Here's how the part is built. I have some questions about the finished solid (model axes, mm). Face numbers are marked on the shaded views. Round coordinates to 2 decimals unless told otherwise and drop trailing zeros. Loops run counter-clockwise (first coordinate to the right, second up) from the corner with the lowest first, then second, coordinate; pieces in that order, holes last. Notation, with made-up numbers: M 67,-23.75 L 100,-23.75 A32 ccw 100,13.25 Z; hole C 30.5,38 d10. An arc over 180 degrees is marked long. Answer as a JSON object with one key per item and string values.
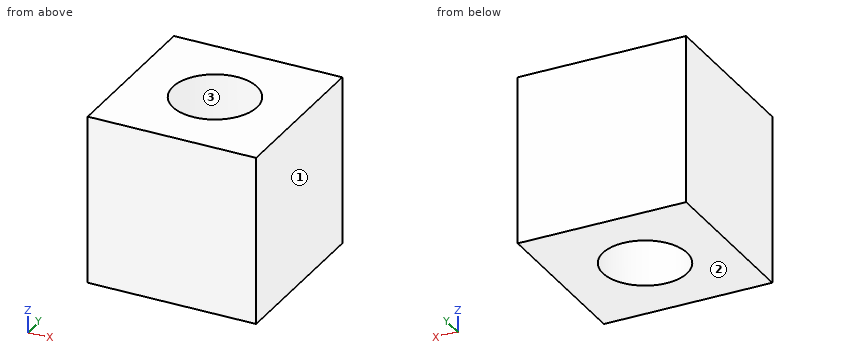
Autodesk Fusion 360 part; units mm, degrees
sketch "WCS Profiles" plane through (0, 0, 0) normal (0, 0, 1) x (1, 0, 0)
  line L0 (20, 20) -> (-20, 20)
  line L1 (-20, 20) -> (-20, -20)
  line L2 (-20, -20) -> (20, -20)
  line L3 (20, -20) -> (20, 20)
  line L4 (20, 20) -> (-20, -20) construction
  line L5 (-20, 20) -> (20, -20) construction
  circle A0 centre (0, 0) radius 10
  dimension "d14" = 40
  dimension "d15" = 20
extrude "Extrude1" add sketch "WCS Profiles" along normal blind 40
Item 1: We'd pull the mould along X, two halves only. Please class the marked faces 1, 2 and 3: +X half, -X half, draft (parallel to the pull), parting line (faces both ways), or undercut.
Solution:
{"face 1": "+X half", "face 2": "draft", "face 3": "undercut"}
Item 2: I want a section at A-A on y = 0. List the corners of the cut face in (x, z) for me, plus the area to 3 significant figures.
Solution:
{"outline": "M -20,0 L -10,0 L -10,40 L -20,40 Z; M 10,0 L 20,0 L 20,40 L 10,40 Z", "area": "800 mm2"}
Item 3: If I drill on L1, parallel to Y at x = 0, z = 23; L2, parallel to X at y = 1.5, z = 32.5; L3, parallel to X at y = 3.5, z = 5.5, over which ranges is the centre line in solid material (lowest first)? Write a range as from..to.
Solution:
{"L1": "y = -20..-10, 10..20", "L2": "x = -20..-9.89, 9.89..20", "L3": "x = -20..-9.37, 9.37..20"}
Item 4: I want a section at B-B on z = 12. List the corners of the cut face in (x, y) for me.
Solution:
{"outline": "M -20,-20 L 20,-20 L 20,20 L -20,20 Z; hole C 0,0 d20"}
